For this review, take the finished solid that the model builds, in its own axes (mm). A direction names the side the tool comes from. Round coordinates to 2 decimals unless told otherwise and drop trailing zeros. Order: outer loops, then holes, each group sorted by start corner. A loop starts at its lowest first (then second) coordinate and runs counter-clockwise, first axis right, second up. Notation, with made-up numbers: (-27, 54.25) -> (-14, 54.25) arc R19 cw to (-14, 88.25) -> close; hole circle Ø9 at (56.5, 86). An arc over 180 degrees is marked (long way). Use a Markdown table: item, result. Add a question column.
1) Consider section B-B (y = 14). State the section outline as (x, z) points.
2) Machinability: for faces 4 (the face through (72, 0, -61)), 5 (the face through (75, 125, -35)), 6 (the face through (-45, 49, -35)), 7 (the face through (-45, 100, -18)), 8 (the face through (26.348, 125.35, -28.662)), which of the approach directions +Z, -Z, +X, -X, +Y, -Y give a long, thin tool a straight path to every point of the face, cutting with its end or side? Answer none if there is none.
3) Consider section C-C (z = -90.5). State the section outline as (x, y) points, plus the area to 3 significant figures.
4) Consider section A-A (x = -17). State the section outline as (y, z) points.
5) Clearance check with flat-ended pins moving along their axes: P1, Ø24, axis at x = -49, y = 28, coming from the +Z side; P2, Ø8, axis at x = 24, z = -13.5, coming from the -Y side; P3, Ø9, axis at x = -48, z = -61, coming from the +Y side; P4, Ø15, axis at x = -47, y = 67.5, coming from the -Z side. State where each tip first meets the part, or that it passes through.
6) Consider section D-D (z = -103). State the section outline as (x, y) points, plus the area to 3 significant figures.
7) Wall thickness on line 1 along Z through (x, y) = (-47.5, 134); line 2 along Z through (x, y) = (-37.5, 47); line 3 along Y through (x, z) = (-13, -70.5): over which ranges is each line inside the solid? List them lowest first. Write a range as [from, to].
8) Draft analysis for pull direction Z (two halves, no side actions). For faces 1 (the face through (-45, 49, -85)), 2 (the face through (26.7, 125.35, -91.34)), 3 (the face through (200, 76, -59)), state which applies: pulls with the +Z half, pulls with the -Z half, needs draft (parallel to the pull), parting line crosses it, or undercut.
```python
from build123d import *

# Parameters (mm, degrees)
SKETCH_1_W          = 120
SKETCH_1_H          = 150
EXTRUDE_1_DEPTH     = 200
CUT_EXTRUDE_1_DEPTH = 50
EXTRUDE_3_DEPTH     = 30
SKETCH_4_W          = 35
SKETCH_4_H          = 50
EXTRUDE_4_DEPTH     = 30
SKETCH_5_W          = 50
SKETCH_5_H          = 99.5
EXTRUDE_7_DEPTH     = 30


with BuildPart() as part:
    # 草图1 → 凸台-拉伸1 (new body)
    with BuildSketch(Plane(origin=(0, 0, 0), x_dir=(0, 0, -1), z_dir=(1, 0, 0))):
        with Locations((60, 75)):
            Rectangle(SKETCH_1_W, SKETCH_1_H)
    extrude(amount=EXTRUDE_1_DEPTH)

    # 草图2 → 切除-拉伸1 (cut)
    with BuildSketch(Plane(origin=(0, 150, 0), x_dir=(1, 0, 0), z_dir=(0, 1, 0))):
        Polygon((75, 85), (25, 85), (71.650635095, 72.5), align=None)
        Polygon((28.349364905, 97.5), (25, 85), (75, 85), align=None)
        Polygon((25, 85), (0, 85), (0, 35), (46.650635095, 47.5), (50, 35), (100, 35), (100, 85), (75, 85), (71.650635095, 72.5), align=None)
        Polygon((46.650635095, 47.5), (0, 35), (50, 35), align=None)
        Polygon((50, 35), (0, 35), (3.349364905, 22.5), align=None)
    extrude(amount=-CUT_EXTRUDE_1_DEPTH, mode=Mode.SUBTRACT)

    # 草图3 → 凸台-拉伸3 (add)
    with BuildSketch(Plane.ZY):
        Polygon((-35, 100), (-85, 100), (-85, 150), (-120, 150), (-120, 0), (0, 0), (0, 150), (-35, 150), align=None)
    extrude(amount=EXTRUDE_3_DEPTH)

    # 草图4 → 凸台-拉伸4 (add)
    with BuildSketch(Plane.ZY.offset(30)):
        with Locations((-102.5, 125)):
            Rectangle(SKETCH_4_W, SKETCH_4_H)
        with Locations((-17.5, 125)):
            Rectangle(SKETCH_4_W, SKETCH_4_H)
    extrude(amount=EXTRUDE_4_DEPTH)

    # 草图5 → 凸台-拉伸7 (add)
    with BuildSketch(Plane.ZY.offset(30)):
        with Locations((-60, 49.75)):
            Rectangle(SKETCH_5_W, SKETCH_5_H)
    extrude(amount=EXTRUDE_7_DEPTH)


solid = part.part
```
Results list:
| question | item | result |
|---|---|---|
| 1 | outline | (-60, -85) -> (-30, -85) -> (-30, -120) -> (200, -120) -> (200, 0) -> (-30, 0) -> (-30, -35) -> (-60, -35) -> close |
| 2 | face 4 | +Z, -Z, +X, -X, -Y |
| 2 | face 5 | -X, +Y |
| 2 | face 6 | +Z, -X, -Y |
| 2 | face 7 | +Z, -Z, -X, -Y |
| 2 | face 8 | +Y |
| 3 | outline | (-60, 100) -> (-30, 100) -> (-30, 0) -> (200, 0) -> (200, 150) -> (54.47, 150) -> (54.47, 100) -> (26.47, 100) -> (26.47, 150) -> (-60, 150) -> close |
| 3 | area | 34,600 mm2 |
| 4 | outline | (0, -120) -> (150, -120) -> (150, -85) -> (100, -85) -> (100, -35) -> (150, -35) -> (150, 0) -> (0, 0) -> close |
| 5 | P1 | z = -35 |
| 5 | P2 | y = 0 |
| 5 | P3 | y = 99.5 |
| 5 | P4 | z = -85 |
| 6 | outline | (-60, 100) -> (-30, 100) -> (-30, 0) -> (200, 0) -> (200, 150) -> (-60, 150) -> close |
| 6 | area | 36,000 mm2 |
| 7 | line 1 | [-120, -85], [-35, 0] |
| 7 | line 2 | [-85, -35] |
| 7 | line 3 | [0, 100] |
| 8 | face 1 | pulls with the -Z half |
| 8 | face 2 | undercut |
| 8 | face 3 | needs draft |
